Verification items for the finished model (mm, model axes). A direction names the side the tool comes from. Coordinates: 2 decimals unless noted, no trailing zeros. Order: outer loops, then holes, each group sorted by start corner. A loop starts at its lowest first (then second) coordinate and runs counter-clockwise, first axis right, second up. Notation, with made-up numbers: M 6,-6 L 46,-6 A22 cw 46,6 Z; hole C 41,72 d4. An arc over 180 degrees is marked long. Return JSON: item names as keys, results as strings.
```python
from build123d import *

# Parameters (mm, degrees)
SKETCH1_W           = 50
SKETCH1_H           = 40
SKETCH1_R           = 3
BOSS_EXTRUDE1_DEPTH = 15
SWEEP1_START        = -20
SWEEP1_DEPTH        = 40
FILLET1_R           = 15
SKETCH3_R           = 3
CUT_EXTRUDE1_DEPTH  = 220.951933549
FILLET2_R           = 10


# Read off the part's stored shape, not the designer's step: Sweep1
with BuildPart() as part:
    # Sketch1 → Boss-Extrude1 (new body)
    with BuildSketch(Plane(origin=(0, 0, 0), x_dir=(1, 0, 0), z_dir=(0, 1, 0))):
        Rectangle(SKETCH1_W, SKETCH1_H)
        with Locations(Location((0, 0, 0), (0, 0, 270))):
            Circle(SKETCH1_R, mode=Mode.SUBTRACT)
    extrude(amount=BOSS_EXTRUDE1_DEPTH)

    # Sweep1 outline → Sweep1 (add)
    with BuildSketch(Plane.XY.offset(SWEEP1_START)):
        Polygon((123.881139344, -76.004182722), (123.881139344, -146.347204208), (137.976528655, -141.216902058), (137.976528655, -71.559923544), (95.277055769, -10.578756452), (25, 15), (25, 0), (86.279911141, -22.304063614), align=None)
    extrude(amount=SWEEP1_DEPTH)

    # Fillet1
    fillet1_edges = [part.edges().sort_by_distance(p)[0] for p in [
        (-25, 7.5, 20),
        (-25, 7.5, -20),
    ]]
    fillet(fillet1_edges, radius=FILLET1_R)

    # Sketch3 → Cut-Extrude1 (cut, through all)
    with BuildSketch(Plane(origin=(137.976528655, 0, 0), x_dir=(0, 0, -1), z_dir=(1, 0, 0))):
        with Locations(Location((0, -106.559923544, 0), (0, 0, 90))):
            Circle(SKETCH3_R)
        with Locations(Location((0, -87.559923544, 0), (0, 0, 90))):
            Circle(SKETCH3_R)
        with Locations(Location((0, -126.559923544, 0), (0, 0, 90))):
            Circle(SKETCH3_R)
    extrude(amount=-CUT_EXTRUDE1_DEPTH, mode=Mode.SUBTRACT)

    # Fillet2
    fillet2_edges = [part.edges().sort_by_distance(p)[0] for p in [
        (123.881139344, -146.347204208, 0),
        (137.976528655, -71.559923544, 0),
        (123.881139344, -76.004182722, 0),
        (95.277055769, -10.578756452, 0),
        (86.279911141, -22.304063614, 0),
        (25, 15, 0),
        (25, 0, 0),
    ]]
    fillet(fillet2_edges, radius=FILLET2_R)


solid = part.part
```
Q1. Draft check along Y on faces 1 (the face through (104.84, -48.81, -0.28)), 2 (the face through (59.95, 2.28, -0.28)), 3 (the face through (131.028, -129.557, 0.132)), 4 (the face through (137.977, -108, -5)). Enter one of: pulls with the +Y half, pulls with the -Y half, needs draft (parallel to the pull), parting line crosses it, or undercut.
Values:
{"face 1": "pulls with the -Y half", "face 2": "pulls with the +Y half", "face 3": "undercut", "face 4": "needs draft"}
Q2. Cross-section at A-A, the plane x = 0. Record the boundary of the cut face in (y, z), and give its area (3 significant figures).
Values:
{"outline": "M 0,-20 L 15,-20 L 15,-3 L 0,-3 Z; M 0,3 L 15,3 L 15,20 L 0,20 Z", "area": "510 mm^2"}
Q3. Material ranges on line 1 along Y through (x, z) = (14.5, 12); line 2 along X through (y, z) = (-120, 17.5); line 3 along Y through (x, z) = (68, -16), recorded low to high.
Values:
{"line 1": "0 to 15", "line 2": "123.88 to 137.98", "line 3": "-15.65 to -0.65"}
Q4. Cross-section at C-C, the plane z = -9. Record the boundary of the cut face in (x, y), and give its area (3 significant figures).
Values:
{"outline": "M -24.46,0 L 23.24,0 A10 cw 26.66,-0.6 L 83.32,-21.23 A10 cw 88.09,-24.89 L 122.07,-73.42 A10 cw 123.88,-79.16 L 123.88,-132.07 A10 ccw 137.3,-141.46 L 137.98,-141.22 L 137.98,-74.71 A10 ccw 136.17,-68.98 L 97.09,-13.16 A10 ccw 92.31,-9.5 L 26.66,14.4 A10 ccw 23.24,15 L -24.46,15 Z", "area": "3,660 mm^2"}
Q5. Cross-section at B-B, the plane z = 0. State how many separate pieces and enclosed holes the cut face has, and give its area (3 significant figures).
Values:
{"separate pieces": "5", "enclosed holes": "0", "area": "3,320 mm^2"}
Q6. Tool access check on faces 5 (the face through (4, 0, 0)), 6 (the face through (137.501, -71.665, 0.28)). Record the directions out of +Z, -Z, +X, -X, +Y, -Y that give a thin tool (end or side, any length) a straight path to the whole face; none if there is none.
Values:
{"face 5": "+Z, -Z, -X, -Y", "face 6": "+Z, -Z, +X, +Y"}
Q7. Cross-section at D-D, the plane x = 50. Record the boundary of the cut face in (y, z), and give its area (3 significant figures).
Values:
{"outline": "M -9.1,-20 L 5.9,-20 L 5.9,20 L -9.1,20 Z", "area": "600 mm^2"}
Q8. Go/stop test with flat-tipped pins: pin 1 (2 mm diameter, centred on x = 48.5, z = 8, fed in from -Y); pin 2 (20 mm diameter, centred on y = -103, z = 7.5, fed in from -X); pin 3 (10 mm diameter, centred on x = 37, z = -10.5, fed in from +Y). Record where each tip stops, or that it passes through.
Values:
{"pin 1": "y = -8.92", "pin 2": "x = 123.88", "pin 3": "y = 12.45"}
